from build123d import *

# Parameters (mm, degrees)
SKETCH_W        = 59.8
SKETCH_H        = 10
SKETCH_W_2      = 10
SKETCH_H_2      = 69.8
PAD_DEPTH       = 10
SKETCH001_R     = 2
SKETCH001_R_2   = 15
POCKET_DEPTH    = 10.001
SKETCH002_R     = 11.5
POCKET001_DEPTH = 10.001


with BuildPart() as part:
    # Sketch → Pad (new body)
    with BuildSketch(Plane.XZ):
        Polygon((0, 0), (0, 30.73), (-10, 30.73), (-10, 80.93), (0, 80.93), (0, 140.1), (-10, 140.1), (-10, 190.1), (0, 190.1), (0, 207.8), (400, 207.8), (400, 190.1), (410, 190.1), (410, 140.1), (400, 140.1), (400, 80.93), (410, 80.93), (410, 30.73), (400, 30.73), (400, 0), align=None)
        with Locations((80.2, 90)):
            Rectangle(SKETCH_W, SKETCH_H, mode=Mode.SUBTRACT)
        with Locations((200, 90)):
            Rectangle(SKETCH_W, SKETCH_H, mode=Mode.SUBTRACT)
        with Locations((319.8, 90)):
            Rectangle(SKETCH_W, SKETCH_H, mode=Mode.SUBTRACT)
        with Locations((165, 152.5)):
            Rectangle(SKETCH_W_2, SKETCH_H_2, mode=Mode.SUBTRACT)
    extrude(amount=PAD_DEPTH)

    # Sketch001 → Pocket (cut, through all)
    with BuildSketch(Plane.XZ):
        with Locations((113, 140.6)):
            Circle(SKETCH001_R)
        with Locations((147, 140.6)):
            Circle(SKETCH001_R)
        with Locations((147, 113.4)):
            Circle(SKETCH001_R)
        with Locations((113, 113.4)):
            Circle(SKETCH001_R)
        with Locations((130, 127)):
            Circle(SKETCH001_R_2)
    extrude(amount=POCKET_DEPTH, mode=Mode.SUBTRACT)

    # Sketch002 → Pocket001 (cut, through all)
    with BuildSketch(Plane.XZ):
        with Locations((80, 170)):
            Circle(SKETCH002_R)
    extrude(amount=POCKET001_DEPTH, mode=Mode.SUBTRACT)


solid = part.part
Input: part model. Units: mm. Frame: model coordinates. A direction names the side the tool comes from. Give positions to 0.01 mm unless a question says otherwise; leave off trailing zeros. Order: outer loops, then holes, each group sorted by start corner. A loop starts at its lowest first (then second) coordinate and runs counter-clockwise, first axis right, second up. Notation, with made-up numbers: M 7,-20 L 50,-20 A21 cw 50,8 Z; hole C 50,31.25 d9. An arc over 180 degrees is marked long. Answer as a JSON object with one key per item and string values.
1. First-contact query: P1, Ø3.5, axis at x = 113, z = 140.6, coming from the -Y side; P2, Ø5, axis at x = 404.5, y = -7.5, coming from the -Z side; P3, Ø3, axis at x = -3.5, y = -5.5, coming from the +Z side; P4, Ø5, axis at y = -5, z = 195.5, coming from the -X side. Flat tips, straight axial feed; report the tip coordinate or a pass-through.
Result sheet:
{"P1": "through", "P2": "z = 30.73", "P3": "z = 190.1", "P4": "x = 0"}
2. Cut plane C-C, the plane x = 80. Output: boundary loops of the cut face in (y, z).
Result sheet:
{"outline": "M -10,0 L 0,0 L 0,85 L -10,85 Z; M -10,95 L 0,95 L 0,158.5 L -10,158.5 Z; M -10,181.5 L 0,181.5 L 0,207.8 L -10,207.8 Z"}
3. Cut plane B-B, the plane z = 170. Output: boundary loops of the cut face in (x, y).
Result sheet:
{"outline": "M -10,-10 L 68.5,-10 L 68.5,0 L -10,0 Z; M 91.5,-10 L 160,-10 L 160,0 L 91.5,0 Z; M 170,-10 L 410,-10 L 410,0 L 170,0 Z"}
4. Cut plane A-A, the plane x = 206. Output: boundary loops of the cut face in (y, z), and give its area (3 significant figures).
Result sheet:
{"outline": "M -10,0 L 0,0 L 0,85 L -10,85 Z; M -10,95 L 0,95 L 0,207.8 L -10,207.8 Z", "area": "1,980 mm²"}
5. Cut plane D-D, the plane y = -7. State how many separate pieces and enclosed holes the cut face has, and give its area (3 significant figures).
Result sheet:
{"separate pieces": "1", "enclosed holes": "10", "area": "81,500 mm²"}
6. Reachability of faces 1 (the flat face through (-5, -5, 30.73)), 2 (the flat face through (349.7, -5, 90)), 3 (the flat face through (-5, -5, 80.93)) from +Z, -Z, +X, -X, +Y, -Y: full face, straight path, thin tool, end or side. Return the list, or none.
Result sheet:
{"face 1": "-Z, -X, +Y, -Y", "face 2": "+Y, -Y", "face 3": "-X, +Y, -Y"}
7. Pull-direction query (Z, two-part tool) for faces 4 (the flat face through (-10, -5, 165)), 5 (the flat face through (405, -5, 80.93)), 6 (the flat face through (197, -5, 207.8)); classes: +Z half, -Z half, draft (parallel to the pull), parting line (faces both ways), or undercut.
Result sheet:
{"face 4": "draft", "face 5": "undercut", "face 6": "+Z half"}
8. Ray query, line 1 (X direction, y = -3, z = 127); line 2 (Z direction, x = 80, y = -6.5); line 3 (Z direction, x = 113, y = -7.5). Return the intervals inside material, ascending. Write a range as [from, to].
Result sheet:
{"line 1": "[0, 115], [145, 160], [170, 400]", "line 2": "[0, 85], [95, 158.5], [181.5, 207.8]", "line 3": "[0, 111.4], [115.4, 138.6], [142.6, 207.8]"}
